from build123d import *

# Parameters (mm, degrees)
BOSS_EXTRUDE1_DEPTH = 40
SKETCH2_R           = 1.55
CUT_EXTRUDE1_DEPTH  = 52.23475383
CUT_EXTRUDE2_DEPTH  = 7
SKETCH4_R           = 2.5
BOSS_EXTRUDE2_DEPTH = 7
CHAMFER1_SIZE       = 0.5
CUT_EXTRUDE3_DEPTH  = 5
CUT_EXTRUDE4_DEPTH  = 5


with BuildPart() as part:
    # Sketch1 → Boss-Extrude1 (new body)
    with BuildSketch(Plane.XY):
        Polygon((16, 0), (0, 0), (0, 20), (25, 20), (25, 10), (16, 10), align=None)
    extrude(amount=BOSS_EXTRUDE1_DEPTH)

    # Sketch2 → Cut-Extrude1 (cut, through all)
    with BuildSketch(Plane(origin=(0, 20, 0), x_dir=(1, 0, 0), z_dir=(0, 1, 0))):
        with Locations(Location((4.5, -10, 0), (0, 0, 270))):
            Circle(SKETCH2_R)
        with Locations(Location((20.5, -10, 0), (0, 0, 270))):
            Circle(SKETCH2_R)
        with Locations(Location((4.5, -30, 0), (0, 0, 270))):
            Circle(SKETCH2_R)
        with Locations(Location((20.5, -30, 0), (0, 0, 270))):
            Circle(SKETCH2_R)
    extrude(amount=-CUT_EXTRUDE1_DEPTH, mode=Mode.SUBTRACT)

    # Sketch3 → Cut-Extrude2 (cut)
    with BuildSketch(Plane(origin=(16, 0, 0), x_dir=(0, 0, -1), z_dir=(1, 0, 0))):
        with BuildLine():
            Line((-40, 5), (-34.186947262, 5))
            ThreePointArc((-34.186947262, 5), (-30.77376681, 5.710822798), (-27.928110681, 7.725099602))
            ThreePointArc((-27.928110681, 7.725099602), (-21.078030656, 5.78622927), (-26.65147843, 1.356839422))
            ThreePointArc((-26.65147843, 1.356839422), (-30.592126256, 2.659238759), (-34.718950561, 3.1))
            Line((-34.718950561, 3.1), (-40, 3.1))
            Line((-40, 3.1), (-40, 5))
        make_face()
        with BuildLine():
            Line((0, 5), (-5.813052738, 5))
            ThreePointArc((-5.813052738, 5), (-9.22623319, 5.710822798), (-12.071889319, 7.725099602))
            ThreePointArc((-12.071889319, 7.725099602), (-18.921969344, 5.78622927), (-13.34852157, 1.356839422))
            ThreePointArc((-13.34852157, 1.356839422), (-9.407873744, 2.659238759), (-5.281049439, 3.1))
            Line((-5.281049439, 3.1), (0, 3.1))
            Line((0, 3.1), (0, 5))
        make_face()
    extrude(amount=-CUT_EXTRUDE2_DEPTH, mode=Mode.SUBTRACT)

    # Sketch4 → Boss-Extrude2 (add)
    with BuildSketch(Plane(origin=(9, 0, 0), x_dir=(0, 0, -1), z_dir=(1, 0, 0))):
        with Locations((-25, 5)):
            Circle(SKETCH4_R)
        with Locations((-15, 5)):
            Circle(SKETCH4_R)
    extrude(amount=BOSS_EXTRUDE2_DEPTH)

    # Chamfer1
    chamfer1_edges = [part.edges().sort_by_distance(p)[0] for p in [
        (16, 5, 27.5),
        (16, 5, 17.5),
    ]]
    chamfer(chamfer1_edges, length=CHAMFER1_SIZE)

    # Sketch5 → Cut-Extrude3 (cut)
    with BuildSketch(Plane.XZ):
        Polygon((7.249630657, 11.5875), (4.5, 13.175), (1.750369343, 11.5875), (1.750369343, 8.4125), (4.5, 6.825), (7.249630657, 8.4125), align=None)
        Polygon((7.249630657, 31.5875), (4.5, 33.175), (1.750369343, 31.5875), (1.750369343, 28.4125), (4.5, 26.825), (7.249630657, 28.4125), align=None)
    extrude(amount=-CUT_EXTRUDE3_DEPTH, mode=Mode.SUBTRACT)

    # Sketch6 → Cut-Extrude4 (cut)
    with BuildSketch(Plane.XZ.offset(-10)):
        Polygon((23.249630657, 11.5875), (20.5, 13.175), (17.750369343, 11.5875), (17.750369343, 8.4125), (20.5, 6.825), (23.249630657, 8.4125), align=None)
        Polygon((23.249630657, 28.4125), (23.249630657, 31.5875), (20.5, 33.175), (17.750369343, 31.5875), (17.750369343, 28.4125), (20.5, 26.825), align=None)
    extrude(amount=-CUT_EXTRUDE4_DEPTH, mode=Mode.SUBTRACT)


solid = part.part
Read the model definition and answer for the solid it produces. Units are mm, in the model's axes. A direction names the side the tool comes from. Round coordinates to 2 decimals unless told otherwise and drop trailing zeros. Write each loop counter-clockwise with the first axis right and the second up, starting at its lowest first coordinate (ties: lowest second). Pieces come first, ordered by that corner, then holes. Notation, with made-up numbers: M 26,71 L 71,71 A17 cw 71,104 Z; hole C -13.75,38 d2. An arc over 180 degrees is marked long. Use a Markdown table: item, result.
1) A tool of negligible diameter and unlimited length cuts with its end or side. For faces 1 (the flat face through (13, 5, 3)), 2 (the flat face through (21.86, 12.46, 27.61)), 3 (the cylindrical face through (22.037, 17.535, 9.798)), 4 (the cylindrical face through (12.549, 2.647, 9.465)), from which of +Z, -Z, +X, -X, +Y, -Y can it reach the whole face along a straight path? Write none if from no direction.
Answers follow:
| item | result |
|---|---|
| face 1 | -Z, +X |
| face 2 | -Y |
| face 3 | +Y, -Y |
| face 4 | +X |
2) The part is cut by section C-C (y = 11.5). Give the number of separate pieces and of enclosed holes in the cut face, plus the area to 3 significant figures.
Answers follow:
| item | result |
|---|---|
| separate pieces | 1 |
| enclosed holes | 4 |
| area | 933 mm2 |
3) The part is cut by section D-D (y = 9.5). Write down the section's boundary in (x, z), plus the area to 3 significant figures.
Answers follow:
| item | result |
|---|---|
| outline | M 0,0 L 16,0 L 16,40 L 0,40 Z; hole C 4.5,10 d3.1; hole C 4.5,30 d3.1 |
| area | 625 mm2 |
4) Straight lines are drawn through the part: line 1 along X through (y, z) = (16.75, 10); line 2 along Y through (x, z) = (13.75, 15); line 3 along X through (y, z) = (12.5, 10). For each, find the intervals that lie inside material, in ascending order. Write a range as [from, to].
Answers follow:
| item | result |
|---|---|
| line 1 | x = [0, 2.95], [6.05, 18.95], [22.05, 25] |
| line 2 | y = [0, 1], [2.5, 7.5], [9, 20] |
| line 3 | x = [0, 2.95], [6.05, 17.75], [23.25, 25] |
5) The part is cut by section A-A (x = 11). Write down the section's boundary in (y, z).
Answers follow:
| item | result |
|---|---|
| outline | M 0,0 L 3.1,0 L 3.1,5.28 A19.54 ccw 1.36,13.35 A4 cw long 7.73,12.07 A8.55 ccw 5,5.81 L 5,0 L 20,0 L 20,40 L 5,40 L 5,34.19 A8.55 ccw 7.73,27.93 A4 cw long 1.36,26.65 A19.54 ccw 3.1,34.72 L 3.1,40 L 0,40 Z; C 5,15 d5; C 5,25 d5 |
6) For a pull along X with two mould halves and no side action, classify faces 5 (the flat face through (9, 4, 28)), 6 (the flat face through (5.86, 2.46, 7.61)), 7 (the flat face through (13, 5, 37)) as pulls with the +X half, pulls with the -X half, needs draft (parallel to the pull), parting line crosses it, or undercut.
Answers follow:
| item | result |
|---|---|
| face 5 | pulls with the +X half |
| face 6 | undercut |
| face 7 | needs draft |
7) Flat-ended cylindrical pins translate along their axes: pin 1 (2 mm diameter, centred on x = 19, y = 8.5, fed in from +Z); pin 2 (4.5 mm diameter, centred on y = 5.5, z = 25, fed in from +X); pin 3 (4.5 mm diameter, centred on x = 21, z = 30.5, fed in from -Y); pin 4 (3.5 mm diameter, centred on x = 4.5, z = 10, fed in from -Y). Find the tip coordinate at first contact, or state that the pin passes through.
Answers follow:
| item | result |
|---|---|
| pin 1 | passes through |
| pin 2 | stops at x = 16 |
| pin 3 | stops at y = 10 |
| pin 4 | stops at y = 5 |
8) The part is cut by section B-B (z = 10). Write down the section's boundary in (x, y).
Answers follow:
| item | result |
|---|---|
| outline | M 0,0 L 1.75,0 L 1.75,5 L 2.95,5 L 2.95,20 L 0,20 Z; M 6.05,5 L 7.25,5 L 7.25,0 L 16,0 L 16,2.52 L 9,2.52 L 9,6.1 L 16,6.1 L 16,10 L 17.75,10 L 17.75,15 L 18.95,15 L 18.95,20 L 6.05,20 Z; M 22.05,15 L 23.25,15 L 23.25,10 L 25,10 L 25,20 L 22.05,20 Z |
